from build123d import *

# Parameters (mm, degrees)
BOSS_EXTRUDE1_DEPTH            = 118.4275
CUT_EXTRUDE1_REACH             = 138.757
SKETCH3_R                      = 3.96875
SKETCH3_R_2                    = 1.5875
CUT_EXTRUDE1_DIRECTION_2_REACH = 138.757
SKETCH4_R                      = 4.7625
CUT_EXTRUDE2_DEPTH             = 6.35


with BuildPart() as part:
    # Sketch2 → Boss-Extrude1 (new body)
    with BuildSketch(Plane(origin=(0, 0, 0), x_dir=(0, 0, -1), z_dir=(1, 0, 0))):
        Polygon((0, -25.4), (0, 25.4), (-63.5, 25.4), (-63.5, 16.51), (-6.35, 16.51), (-6.35, -16.51), (-63.5, -16.51), (-63.5, -25.4), align=None)
    extrude(amount=BOSS_EXTRUDE1_DEPTH)

    # Cut-Extrude1: up to this face of the body (flat: up to its plane)
    cut_extrude1_end = Plane(part.part.faces().sort_by_distance((59.21375, -25.4, 31.75))[0])
    # Sketch3 → Cut-Extrude1 (cut, up to the picked face)
    with BuildSketch(Plane(origin=(0, 0, 0), x_dir=(1, 0, 0), z_dir=(0, 1, 0)), mode=Mode.PRIVATE) as cut_extrude1_sk1:
        with Locations(Location((7.9375, -19.05, 0), (0, 0, 270))):
            Circle(SKETCH3_R)
    cut_extrude1_tool1 = split(extrude(cut_extrude1_sk1.sketch, amount=-CUT_EXTRUDE1_REACH, mode=Mode.PRIVATE), bisect_by=cut_extrude1_end, keep=Keep.BOTH, mode=Mode.PRIVATE)
    # Sketch3 → Cut-Extrude1 (cut, up to the picked face)
    with BuildSketch(Plane(origin=(0, 0, 0), x_dir=(1, 0, 0), z_dir=(0, 1, 0)), mode=Mode.PRIVATE) as cut_extrude1_sk2:
        with Locations(Location((110.49, -19.05, 0), (0, 0, 270))):
            Circle(SKETCH3_R)
    cut_extrude1_tool2 = split(extrude(cut_extrude1_sk2.sketch, amount=-CUT_EXTRUDE1_REACH, mode=Mode.PRIVATE), bisect_by=cut_extrude1_end, keep=Keep.BOTH, mode=Mode.PRIVATE)
    # Sketch3 → Cut-Extrude1 (cut, up to the picked face)
    with BuildSketch(Plane(origin=(0, 0, 0), x_dir=(1, 0, 0), z_dir=(0, 1, 0)), mode=Mode.PRIVATE) as cut_extrude1_sk3:
        with Locations(Location((37.1475, -14.605, 0), (0, 0, 270))):
            Circle(SKETCH3_R_2)
    cut_extrude1_tool3 = split(extrude(cut_extrude1_sk3.sketch, amount=-CUT_EXTRUDE1_REACH, mode=Mode.PRIVATE), bisect_by=cut_extrude1_end, keep=Keep.BOTH, mode=Mode.PRIVATE)
    # Sketch3 → Cut-Extrude1 (cut, up to the picked face)
    with BuildSketch(Plane(origin=(0, 0, 0), x_dir=(1, 0, 0), z_dir=(0, 1, 0)), mode=Mode.PRIVATE) as cut_extrude1_sk4:
        with Locations(Location((43.4975, -14.605, 0), (0, 0, 270))):
            Circle(SKETCH3_R_2)
    cut_extrude1_tool4 = split(extrude(cut_extrude1_sk4.sketch, amount=-CUT_EXTRUDE1_REACH, mode=Mode.PRIVATE), bisect_by=cut_extrude1_end, keep=Keep.BOTH, mode=Mode.PRIVATE)
    # Sketch3 → Cut-Extrude1 (cut, up to the picked face)
    with BuildSketch(Plane(origin=(0, 0, 0), x_dir=(1, 0, 0), z_dir=(0, 1, 0)), mode=Mode.PRIVATE) as cut_extrude1_sk5:
        with BuildLine():
            Line((15.875, -19.05), (102.5525, -19.05))
            ThreePointArc((102.5525, -19.05), (110.49, -26.9875), (118.4275, -19.05))
            Line((118.4275, -19.05), (118.4275, -63.5))
            Line((118.4275, -63.5), (0, -63.5))
            Line((0, -63.5), (0, -19.05))
            ThreePointArc((0, -19.05), (7.9375, -26.9875), (15.875, -19.05))
        make_face()
    cut_extrude1_tool5 = split(extrude(cut_extrude1_sk5.sketch, amount=-CUT_EXTRUDE1_REACH, mode=Mode.PRIVATE), bisect_by=cut_extrude1_end, keep=Keep.BOTH, mode=Mode.PRIVATE)
    add(cut_extrude1_tool1.solids().sort_by(Axis((7.9375, 0, 19.05), (0, -1, 0)))[0], mode=Mode.SUBTRACT)
    add(cut_extrude1_tool2.solids().sort_by(Axis((110.49, 0, 19.05), (0, -1, 0)))[0], mode=Mode.SUBTRACT)
    add(cut_extrude1_tool3.solids().sort_by(Axis((37.1475, 0, 14.605), (0, -1, 0)))[0], mode=Mode.SUBTRACT)
    add(cut_extrude1_tool4.solids().sort_by(Axis((43.4975, 0, 14.605), (0, -1, 0)))[0], mode=Mode.SUBTRACT)
    add(cut_extrude1_tool5.solids().sort_by(Axis((59.21375, 0, 42.011703), (0, -1, 0)))[0], mode=Mode.SUBTRACT)

    # Cut-Extrude1 direction 2: up to this face of the body (flat: up to its plane)
    cut_extrude1_direction_2_end = Plane(part.part.faces().sort_by_distance((59.21375, 25.4, 31.75))[0])
    # Sketch3 → Cut-Extrude1 direction 2 (cut, up to the picked face)
    with BuildSketch(Plane(origin=(0, 0, 0), x_dir=(1, 0, 0), z_dir=(0, 1, 0)), mode=Mode.PRIVATE) as cut_extrude1_direction_2_sk1:
        with Locations(Location((7.9375, -19.05, 0), (0, 0, 270))):
            Circle(SKETCH3_R)
    cut_extrude1_direction_2_tool1 = split(extrude(cut_extrude1_direction_2_sk1.sketch, amount=CUT_EXTRUDE1_DIRECTION_2_REACH, mode=Mode.PRIVATE), bisect_by=cut_extrude1_direction_2_end, keep=Keep.BOTH, mode=Mode.PRIVATE)
    # Sketch3 → Cut-Extrude1 direction 2 (cut, up to the picked face)
    with BuildSketch(Plane(origin=(0, 0, 0), x_dir=(1, 0, 0), z_dir=(0, 1, 0)), mode=Mode.PRIVATE) as cut_extrude1_direction_2_sk2:
        with Locations(Location((110.49, -19.05, 0), (0, 0, 270))):
            Circle(SKETCH3_R)
    cut_extrude1_direction_2_tool2 = split(extrude(cut_extrude1_direction_2_sk2.sketch, amount=CUT_EXTRUDE1_DIRECTION_2_REACH, mode=Mode.PRIVATE), bisect_by=cut_extrude1_direction_2_end, keep=Keep.BOTH, mode=Mode.PRIVATE)
    # Sketch3 → Cut-Extrude1 direction 2 (cut, up to the picked face)
    with BuildSketch(Plane(origin=(0, 0, 0), x_dir=(1, 0, 0), z_dir=(0, 1, 0)), mode=Mode.PRIVATE) as cut_extrude1_direction_2_sk3:
        with Locations(Location((37.1475, -14.605, 0), (0, 0, 270))):
            Circle(SKETCH3_R_2)
    cut_extrude1_direction_2_tool3 = split(extrude(cut_extrude1_direction_2_sk3.sketch, amount=CUT_EXTRUDE1_DIRECTION_2_REACH, mode=Mode.PRIVATE), bisect_by=cut_extrude1_direction_2_end, keep=Keep.BOTH, mode=Mode.PRIVATE)
    # Sketch3 → Cut-Extrude1 direction 2 (cut, up to the picked face)
    with BuildSketch(Plane(origin=(0, 0, 0), x_dir=(1, 0, 0), z_dir=(0, 1, 0)), mode=Mode.PRIVATE) as cut_extrude1_direction_2_sk4:
        with Locations(Location((43.4975, -14.605, 0), (0, 0, 270))):
            Circle(SKETCH3_R_2)
    cut_extrude1_direction_2_tool4 = split(extrude(cut_extrude1_direction_2_sk4.sketch, amount=CUT_EXTRUDE1_DIRECTION_2_REACH, mode=Mode.PRIVATE), bisect_by=cut_extrude1_direction_2_end, keep=Keep.BOTH, mode=Mode.PRIVATE)
    # Sketch3 → Cut-Extrude1 direction 2 (cut, up to the picked face)
    with BuildSketch(Plane(origin=(0, 0, 0), x_dir=(1, 0, 0), z_dir=(0, 1, 0)), mode=Mode.PRIVATE) as cut_extrude1_direction_2_sk5:
        with BuildLine():
            Line((15.875, -19.05), (102.5525, -19.05))
            ThreePointArc((102.5525, -19.05), (110.49, -26.9875), (118.4275, -19.05))
            Line((118.4275, -19.05), (118.4275, -63.5))
            Line((118.4275, -63.5), (0, -63.5))
            Line((0, -63.5), (0, -19.05))
            ThreePointArc((0, -19.05), (7.9375, -26.9875), (15.875, -19.05))
        make_face()
    cut_extrude1_direction_2_tool5 = split(extrude(cut_extrude1_direction_2_sk5.sketch, amount=CUT_EXTRUDE1_DIRECTION_2_REACH, mode=Mode.PRIVATE), bisect_by=cut_extrude1_direction_2_end, keep=Keep.BOTH, mode=Mode.PRIVATE)
    add(cut_extrude1_direction_2_tool1.solids().sort_by(Axis((7.9375, 0, 19.05), (0, 1, 0)))[0], mode=Mode.SUBTRACT)
    add(cut_extrude1_direction_2_tool2.solids().sort_by(Axis((110.49, 0, 19.05), (0, 1, 0)))[0], mode=Mode.SUBTRACT)
    add(cut_extrude1_direction_2_tool3.solids().sort_by(Axis((37.1475, 0, 14.605), (0, 1, 0)))[0], mode=Mode.SUBTRACT)
    add(cut_extrude1_direction_2_tool4.solids().sort_by(Axis((43.4975, 0, 14.605), (0, 1, 0)))[0], mode=Mode.SUBTRACT)
    add(cut_extrude1_direction_2_tool5.solids().sort_by(Axis((59.21375, 0, 42.011703), (0, 1, 0)))[0], mode=Mode.SUBTRACT)

    # Sketch4 → Cut-Extrude2 (cut)
    with BuildSketch(Plane.XY):
        with Locations(Location((19.05, 0, 0), (0, 0, 180))):
            Circle(SKETCH4_R)
        with Locations(Location((99.3775, 0, 0), (0, 0, 180))):
            Circle(SKETCH4_R)
    extrude(amount=CUT_EXTRUDE2_DEPTH, mode=Mode.SUBTRACT)


solid = part.part
Verification items for the finished model (mm, model axes). A direction names the side the tool comes from. Give positions to 0.01 mm unless a question says otherwise; leave off trailing zeros. Loops run counter-clockwise (first coordinate to the right, second up) from the corner with the lowest first, then second, coordinate; pieces in that order, holes last. Notation, with made-up numbers: (22, 83.25) - (51, 83.25) arc R7 ccw to (51, 92.25) - close; hole circle Ø10 at (35, 60). An arc over 180 degrees is marked (long way). Write item = value, one per line. Start each with the question number.
Q1. Tool access check on faces 4 (the face through (58, 16.51, 12)), 5 (the face through (59, 21, 19.05)), 6 (the face through (36.54, 20.89, 16.07)). Record the directions out of +Z, -Z, +X, -X, +Y, -Y that give a thin tool (end or side, any length) a straight path to the whole face; none if there is none.
Q2. Depth check by flat-ended pin: P1, Ø4.5, axis at x = 74, y = -19.5, coming from the +Z side; P2, Ø11, axis at x = 99.38, y = 0, coming from the +Z side; P3, Ø3, axis at x = 103, y = -19.5, coming from the +Z side. Enter the tip coordinate at first touch or a pass-through.
Q3. Cross-section at A-A, the plane z = 10. Enter the section's corners in (x, y), and give its area (3 significant figures).
Q4. Cross-section at C-C, the plane x = 19.05. Enter the section's corners in (y, z).
Q5. Thickness scan on line 1 (Y direction, x = 85, z = 18.5); line 2 (X direction, y = 19, z = 15); line 3 (X direction, y = -22, z = 14). Record the ranges inside material, lowest first.
Q6. Mould release check, pull along X, two halves, no side actions. Record for faces 1 (the face through (58, 0, 0)), 2 (the face through (118.428, 0, 5)), 3 (the face through (7.763, -20.893, 26.986)): released by +X, released by -X, zero draft, split by the parting line, or undercut.
Q7. Cross-section at B-B, the plane y = 0. State how many separate pieces and enclosed holes the cut face has, and give its area (3 significant figures).
Answer key:
q1.face_4 = +Z, +X, -X
q1.face_5 = +Z, +Y, -Y
q1.face_6 = +Y, -Y
q2.P1 = 19.05
q2.P2 = 6.35
q2.P3 = 24.26
q3.outline = (0, -25.4) - (118.43, -25.4) - (118.43, -16.51) - (0, -16.51) - close; (0, 16.51) - (118.43, 16.51) - (118.43, 25.4) - (0, 25.4) - close
q3.area = 2,110 mm^2
q4.outline = (-25.4, 0) - (-4.76, 0) - (-4.76, 6.35) - (-16.51, 6.35) - (-16.51, 19.05) - (-25.4, 19.05) - close; (4.76, 0) - (25.4, 0) - (25.4, 19.05) - (16.51, 19.05) - (16.51, 6.35) - (4.76, 6.35) - close
q5.line_1 = -25.4 to -16.51, 16.51 to 25.4
q5.line_2 = 0 to 35.61, 38.69 to 41.96, 45.04 to 118.43
q5.line_3 = 0 to 35.68, 38.62 to 42.03, 44.97 to 118.43
q6.face_1 = zero draft
q6.face_2 = released by +X
q6.face_3 = undercut
q7.separate_pieces = 3
q7.enclosed_holes = 0
q7.area = 631 mm^2
